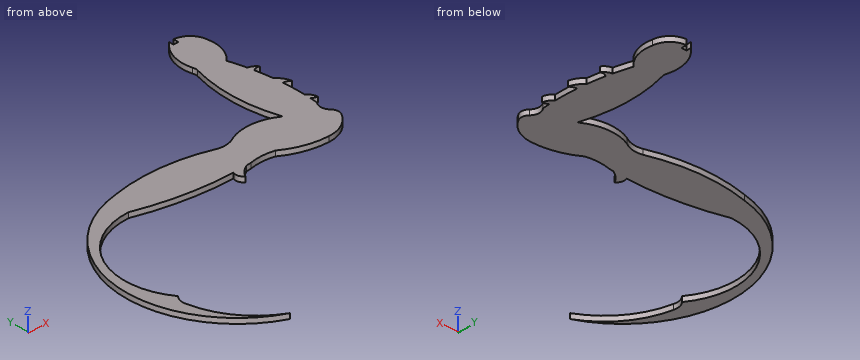
from build123d import *

# Parameters (mm, degrees)
BOSS_EXTRUDE1_DEPTH = 1.524


with BuildPart() as part:
    # Sketch1 → Boss-Extrude1 (new body)
    with BuildSketch(Plane.XY):
        with BuildLine():
            Line((-1.524, 93.996264428), (0, 93.996264428))
            Line((0, 93.996264428), (0, 95.614927588))
            ThreePointArc((0, 95.614927588), (3.693748092, 94.060684173), (5.394313408, 90.431975702))
            ThreePointArc((5.394313408, 90.431975702), (5.083870366, 85.328096728), (2.344513216, 81.010472628))
            ThreePointArc((2.344513216, 81.010472628), (3.08526248, 78.397508533), (3.719210033, 75.756599345))
            ThreePointArc((3.719210033, 75.756599345), (5.090797567, 75.29470873), (6.107013429, 74.264223104))
            ThreePointArc((6.107013429, 74.264223104), (5.043110614, 74.395683401), (4.100454534, 73.885222311))
            ThreePointArc((4.100454534, 73.885222311), (4.539807281, 71.277090284), (4.875594315, 68.653613474))
            ThreePointArc((4.875594315, 68.653613474), (6.349854496, 67.059002397), (7.15480331, 65.042003395))
            ThreePointArc((7.15480331, 65.042003395), (6.204169614, 65.603166167), (5.120829927, 65.815258603))
            ThreePointArc((5.120829927, 65.815258603), (5.25598444, 62.33072683), (5.209157654, 58.843889342))
            ThreePointArc((5.209157654, 58.843889342), (6.301599024, 57.713807832), (6.751402544, 56.207756982))
            ThreePointArc((6.751402544, 56.207756982), (5.901509406, 56.458638265), (5.099422344, 56.835355808))
            ThreePointArc((5.099422344, 56.835355808), (5.010976532, 55.705411647), (4.903376867, 54.577130307))
            ThreePointArc((4.903376867, 54.577130307), (4.160208316, 52.476052404), (5.072854771, 50.442851897))
            ThreePointArc((5.072854771, 50.442851897), (5.82334848, 48.971843275), (5.510783631, 47.350297597))
            ThreePointArc((5.510783631, 47.350297597), (1.996073925, 43.775155466), (-2.817678827, 42.374223627))
            ThreePointArc((-2.817678827, 42.374223627), (-9.49417325, 43.186036631), (-15.638900273, 45.92043747))
            ThreePointArc((-15.638900273, 45.92043747), (-19.39296862, 46.30049438), (-23.12808354, 45.765341186))
            ThreePointArc((-23.12808354, 45.765341186), (-23.817150151, 45.692245813), (-24.506779764, 45.624668263))
            ThreePointArc((-24.506779764, 45.624668263), (-26.42654707, 44.241801226), (-27.879124662, 42.374223627))
            ThreePointArc((-27.879124662, 42.374223627), (-28.871257944, 43.69170684), (-28.707753031, 45.332851748))
            ThreePointArc((-28.707753031, 45.332851748), (-42.992230857, 45.870590172), (-56.993482586, 48.751635021))
            ThreePointArc((-56.993482586, 48.751635021), (-75.256918565, 36.987495898), (-73.1639091, 15.364189619))
            ThreePointArc((-73.1639091, 15.364189619), (-74.068740922, 13.643348437), (-74.042155454, 11.699304143))
            ThreePointArc((-74.042155454, 11.699304143), (-69.240477752, 0.882449229), (-60.077247453, -6.607255003))
            ThreePointArc((-60.077247453, -6.607255003), (-80.312075554, 27.040950348), (-53.970648666, 56.157598868))
            ThreePointArc((-53.970648666, 56.157598868), (-39.168269925, 57.733871806), (-24.506779764, 55.157875102))
            ThreePointArc((-24.506779764, 55.157875102), (-21.512905256, 55.048508832), (-18.750408328, 56.207756982))
            ThreePointArc((-18.750408328, 56.207756982), (-11.598379652, 57.610020261), (-4.659613728, 55.380360214))
            ThreePointArc((-4.659613728, 55.380360214), (-6.824036174, 68.85301684), (-5.055416365, 82.38332301))
            ThreePointArc((-5.055416365, 82.38332301), (-4.963334277, 83.197390982), (-5.135176923, 83.998425237))
            ThreePointArc((-5.135176923, 83.998425237), (-4.912918532, 90.191927066), (-1.524, 95.380770374))
            Line((-1.524, 95.380770374), (-1.524, 93.996264428))
        make_face()
    extrude(amount=BOSS_EXTRUDE1_DEPTH)


solid = part.part
Geometry: final body of the model. Coordinates: model frame, mm. Give positions to 0.01 mm unless a question says otherwise; leave off trailing zeros. Loops run counter-clockwise (first coordinate to the right, second up) from the corner with the lowest first, then second, coordinate; pieces in that order, holes last. Notation, with made-up numbers: M 37.5,-38.5 L 48.5,-38.5 A22 ccw 48.5,-15.5 Z; hole C -6.75,23.5 d8. An arc over 180 degrees is marked long. Put each result on its own line as item: value. Start each with the question number.
1) Cut plane D-D (y = 26). Output: boundary loops of the cut face in (x, z), then the cut area to 3 significant figures.
2) Ray query, line 1 along X through (y, z) = (86, 0.15); line 2 along X through (y, z) = (90, 0.15); line 3 along Y through (x, z) = (-53.5, 1.25). Return the intervals inside material, ascending.
3) Cut plane A-A (x = -68). Output: boundary loops of the cut face in (y, z), then the cut area to 3 significant figures.
4) Cut plane B-B (y = 44). Output: boundary loops of the cut face in (x, z), then the cut area to 3 significant figures.
Verdict:
1. outline: M -80.4,0 L -77.26,0 L -77.26,1.52 L -80.4,1.52 Z
1. area: 4.78 mm2
2. line 1: -5.43 to 5.28
2. line 2: -4.97 to 5.47
2. line 3: 47.8 to 56.27
3. outline: M -1.96,0 L -0.62,0 L -0.62,1.52 L -1.96,1.52 Z; M 45.29,0 L 49.66,0 L 49.66,1.52 L 45.29,1.52 Z
3. area: 8.69 mm2
4. outline: M -73.59,0 L -69.74,0 L -69.74,1.52 L -73.59,1.52 Z; M -28.93,0 L -26.67,0 L -26.67,1.52 L -28.93,1.52 Z; M -11.9,0 L 2.35,0 L 2.35,1.52 L -11.9,1.52 Z
4. area: 31.0 mm2
